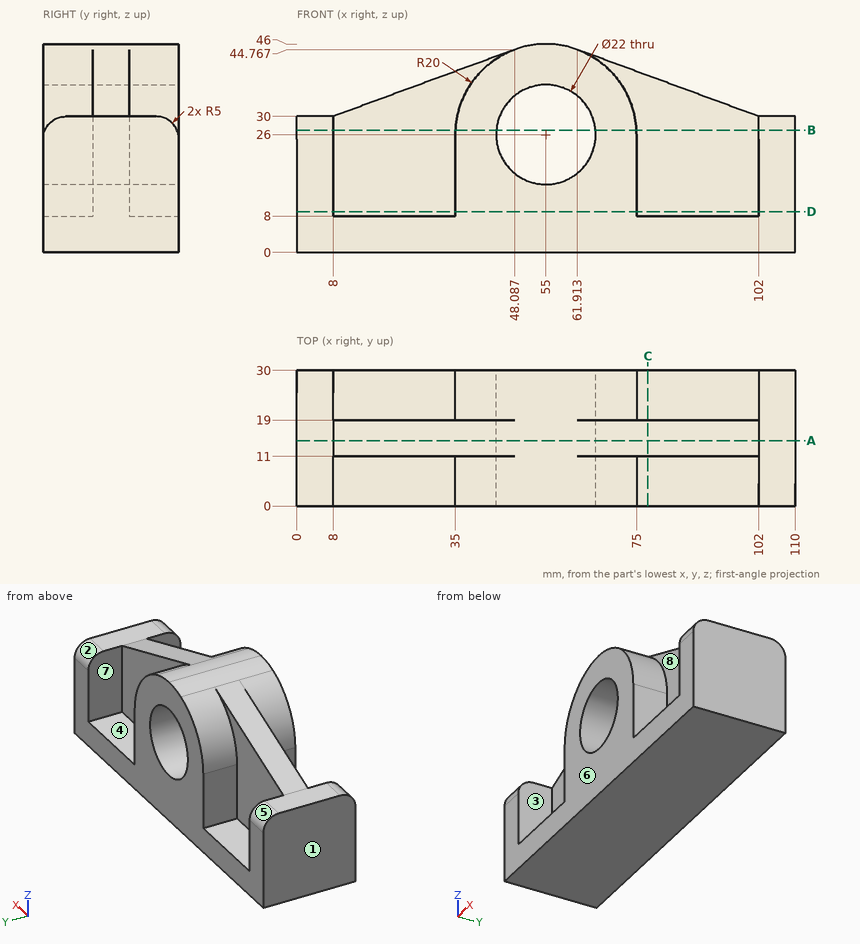
Check sheet for the drawn part. Datum: minimum x, y, z corner. Units: mm. A direction names the side the tool comes from. Coordinates: 2 decimals unless noted, no trailing zeros. Loops run counter-clockwise (first coordinate to the right, second up) from the corner with the lowest first, then second, coordinate; pieces in that order, holes last. Notation, with made-up numbers: M 72,13.25 L 92,13.25 A15 ccw 92,18.25 Z; hole C 89.25,-25.5 d9. An arc over 180 degrees is marked long. Answer as a JSON object with one key per item and string values.
1. Sectioned sample at D-D on z = 9. Record the cut outline in (x, y).
Outcome:
{"outline": "M 0,0 L 8,0 L 8,11 L 35,11 L 35,0 L 75,0 L 75,11 L 102,11 L 102,0 L 110,0 L 110,30 L 102,30 L 102,19 L 75,19 L 75,30 L 35,30 L 35,19 L 8,19 L 8,30 L 0,30 Z"}
2. Sectioned sample at A-A on y = 14.5. Record the cut outline in (x, z).
Outcome:
{"outline": "M 0,0 L 110,0 L 110,30 L 102,30 L 61.91,44.77 A20 ccw 55,46 A20 ccw 48.09,44.77 L 8,30 L 0,30 Z; hole C 55,26 d22"}
3. Access from +Z, -Z, +X, -X, +Y, -Y to the whole of each face (thin tool, end or side, straight path). Record for the marked faces 5, 6, 7 and 8.
Outcome:
{"face 5": "+Z, -X, +Y", "face 6": "+Z, -Z, +X, -X, -Y", "face 7": "+Z, +Y", "face 8": "+Z, -Y"}
4. Sectioned sample at B-B on z = 27. Record the cut outline in (x, y) (1 decimal).
Outcome:
{"outline": "M 0,0.4 L 8,0.4 L 8,11 L 35,11 L 35,0 L 44,0 L 44,30 L 35,30 L 35,19 L 8,19 L 8,29.6 L 0,29.6 Z; M 66,0 L 75,0 L 75,11 L 102,11 L 102,0.4 L 110,0.4 L 110,29.6 L 102,29.6 L 102,19 L 75,19 L 75,30 L 66,30 Z"}
5. Release check for a two-part mould opening along X. For the marked faces 1, 2, 3 and 4 record: pulls with the +X half, pulls with the -X half, needs draft (parallel to the pull), parting line crosses it, or undercut.
Outcome:
{"face 1": "pulls with the -X half", "face 2": "needs draft", "face 3": "undercut", "face 4": "undercut"}
6. Depth check by flat-ended pin: P1, Ø3.5, axis at x = 27, y = 3.5, coming from the +Z side; P2, Ø11, axis at x = 82, z = 18.5, coming from the -Y side; P3, Ø4, axis at x = 4, y = 15, coming from the +Z side. Enter the tip coordinate at first touch or a pass-through.
Outcome:
{"P1": "z = 8", "P2": "y = 11", "P3": "z = 30"}
7. Scan lines: L1, parallel to Z at x = 55, y = 11.75; L2, parallel to X at y = 4.75, z = 25.5; L3, parallel to X at y = 19.5, z = 16 (1 decimal). Record each from-to range of solid material in increasing order. Write a range as from..to.
Outcome:
{"L1": "0..15, 37..46", "L2": "0..8, 35..44.01, 65.99..75, 102..110", "L3": "0..8, 35..50.4, 59.6..75, 102..110"}
8. Sectioned sample at C-C on x = 77.5. Record the cut outline in (y, z) (1 decimal), and give its area (3 significant figures).
Outcome:
{"outline": "M 0,0 L 30,0 L 30,8 L 19,8 L 19,39 L 11,39 L 11,8 L 0,8 Z", "area": "488 mm²"}
